from build123d import *

# Parameters (mm, degrees)
CYLINDER1016_R               = 1.5
CYLINDER1016_DEPTH           = 50
CYLINDER1016_PLACEMENT_ANGLE = 45
CYLINDER1012_R               = 1.5
CYLINDER1012_DEPTH           = 50
CYLINDER1012_PLACEMENT_ANGLE = 135
CYLINDER1014_R               = 1.5
CYLINDER1014_DEPTH           = 50
CYLINDER1017_R               = 1.5
CYLINDER1017_DEPTH           = 50
CYLINDER1017_PLACEMENT_ANGLE = 225
CYLINDER1018_R               = 1.5
CYLINDER1018_DEPTH           = 50
CYLINDER1013_R               = 1.5
CYLINDER1013_DEPTH           = 50
CYLINDER1013_PLACEMENT_ANGLE = 45
CYLINDER1015_R               = 1.5
CYLINDER1015_DEPTH           = 50
CYLINDER1011_R               = 52
CYLINDER1011_DEPTH           = 16
BOX416_W                     = 108
BOX416_H                     = 36
BOX416_DEPTH                 = 16


with BuildPart() as obj1:
    # Cylinder1016 → Cylinder1016 (new body)
    with BuildSketch(Plane.XY):
        Circle(CYLINDER1016_R)
    extrude(amount=CYLINDER1016_DEPTH)


with BuildPart() as obj1_1:
    # Cylinder1016 placement: moved
    add(obj1.part.moved(Location((39.59798, -39.59798, 2))).rotate(Axis((39.59798, -39.59798, 2), (0, 0, 1)), CYLINDER1016_PLACEMENT_ANGLE))


with BuildPart() as obj2:
    # Cylinder1012 → Cylinder1012 (new body)
    with BuildSketch(Plane.XY):
        Circle(CYLINDER1012_R)
    extrude(amount=CYLINDER1012_DEPTH)


with BuildPart() as obj2_1:
    # Cylinder1012 placement: moved
    add(obj2.part.moved(Location((39.59798, 39.59798, 2))).rotate(Axis((39.59798, 39.59798, 2), (0, 0, 1)), CYLINDER1012_PLACEMENT_ANGLE))


with BuildPart() as obj3:
    # Cylinder1014 → Cylinder1014 (new body)
    with BuildSketch(Plane(origin=(0, 56, 2), x_dir=(-1, 0, 0), z_dir=(0, 0, 1))):
        Circle(CYLINDER1014_R)
    extrude(amount=CYLINDER1014_DEPTH)


with BuildPart() as obj4:
    # Cylinder1017 → Cylinder1017 (new body)
    with BuildSketch(Plane.XY):
        Circle(CYLINDER1017_R)
    extrude(amount=CYLINDER1017_DEPTH)


with BuildPart() as obj4_1:
    # Cylinder1017 placement: moved
    add(obj4.part.moved(Location((-39.59798, 39.59798, 2))).rotate(Axis((-39.59798, 39.59798, 2), (0, 0, 1)), CYLINDER1017_PLACEMENT_ANGLE))


with BuildPart() as obj5:
    # Cylinder1018 → Cylinder1018 (new body)
    with BuildSketch(Plane(origin=(-56, 0, 2), x_dir=(0, -1, 0), z_dir=(0, 0, 1))):
        Circle(CYLINDER1018_R)
    extrude(amount=CYLINDER1018_DEPTH)


with BuildPart() as obj6:
    # Cylinder1013 → Cylinder1013 (new body)
    with BuildSketch(Plane.XY):
        Circle(CYLINDER1013_R)
    extrude(amount=CYLINDER1013_DEPTH)


with BuildPart() as obj6_1:
    # Cylinder1013 placement: moved
    add(obj6.part.moved(Location((-39.59798, -39.59798, 2))).rotate(Axis((-39.59798, -39.59798, 2), (0, 0, -1)), CYLINDER1013_PLACEMENT_ANGLE))


with BuildPart() as compound817:
    # Cylinder1015 → Cylinder1015 (new body)
    with BuildSketch(Plane(origin=(0, -56, 2), x_dir=(1, 0, 0), z_dir=(0, 0, 1))):
        Circle(CYLINDER1015_R)
    extrude(amount=CYLINDER1015_DEPTH)

    # Compound817: union obj1, obj2, obj3, obj4, obj5, obj6
    add(obj1_1.part)
    add(obj2_1.part)
    add(obj3.part)
    add(obj4_1.part)
    add(obj5.part)
    add(obj6_1.part)


with BuildPart() as obj7:
    # Cylinder1011 → Cylinder1011 (new body)
    with BuildSketch(Plane.XY.offset(20)):
        Circle(CYLINDER1011_R)
    extrude(amount=CYLINDER1011_DEPTH)


with BuildPart() as cut423:
    # Box416 → Box416 (new body)
    with BuildSketch(Plane(origin=(-54, -53, 20), x_dir=(1, 0, 0), z_dir=(0, 0, 1))):
        with Locations((54, 18)):
            Rectangle(BOX416_W, BOX416_H)
    extrude(amount=BOX416_DEPTH)

    # Cut424: cut obj7
    add(obj7.part, mode=Mode.SUBTRACT)


with BuildPart() as cut423_1:
    # Cut424 placement: moved
    add(cut423.part.moved(Location((0, 0, -10))))

    # Cut423: cut Compound817
    add(compound817.part, mode=Mode.SUBTRACT)


with BuildPart() as cut423_2:
    # Cut423 placement: moved
    add(cut423_1.part.moved(Location((0, 0, 6))))


solid = cut423_2.part
The model under review builds one solid part; all positions refer to its coordinate system, in mm. Coordinates: 2 decimals unless noted, no trailing zeros. Loops run counter-clockwise (first coordinate to the right, second up) from the corner with the lowest first, then second, coordinate; pieces in that order, holes last.
(1) Wall thickness on L1, parallel to X at y = -39.5, z = 23.5; L2, parallel to X at y = -19, z = 18; L3, parallel to X at y = -33.5, z = 18.25: over which ranges is each line inside the solid? List them lowest first.
Determined:
L1: x = -54 to -41.09, -38.1 to -33.82, 33.82 to 38.1, 41.09 to 54
L2: x = -54 to -48.4, 48.4 to 54
L3: x = -54 to -39.77, 39.77 to 54
(2) Consider section A-A, the plane y = -24. Give the boundary of the cut face in (x, z), plus the area to 3 significant figures.
Determined:
outline: (-54, 16) - (-46.13, 16) - (-46.13, 32) - (-54, 32) - close; (46.13, 16) - (54, 16) - (54, 32) - (46.13, 32) - close
area: 252 mm2
(3) Insertion check: P1, Ø2.5, axis at x = 39.6, y = -39.6, coming from the +Z side; P2, Ø1.5, axis at x = -8.5, z = 21.5, coming from the +Y side. Each pin has a flat end and moves straight along its axis. Give the tip position at first contact, or say it passes through.
Determined:
P1: passes through
P2: stops at y = -51.17
(4) Draft analysis for pull direction X (two halves, no side actions). For faces 1 (the flat face through (-13, -51, 32)), 2 (the cylindrical face through (-40.61, -38.49, 23.89)), 3 (the cylindrical face through (38.49, -40.61, 23.89)), 4 (the flat face through (54, -35, 24)), state which applies: +X half, -X half, draft (parallel to the pull), parting line (faces both ways), or undercut.
Determined:
face 1: draft
face 2: undercut
face 3: undercut
face 4: +X half
(5) Consider section B-B, the plane z = 27.25. Give the boundary of the cut face in (x, y), plus the area to 3 significant figures.
Determined:
outline: (-54, -53) - (54, -53) - (54, -17) - (49.14, -17) arc R52 cw to (-49.14, -17) - (-54, -17) - close; hole circle Ø3 at (-39.6, -39.6); hole circle Ø3 at (39.6, -39.6)
area: 1,360 mm2
(6) Consider section C-C, the plane y = -50.5. Give the boundary of the cut face in (x, z), plus the area to 3 significant figures.
Determined:
outline: (-54, 16) - (-12.4, 16) - (-12.4, 32) - (-54, 32) - close; (12.4, 16) - (54, 16) - (54, 32) - (12.4, 32) - close
area: 1,330 mm2
(7) Consider section D-D, the plane x = 5. Give the boundary of the cut face in (y, z), plus the area to 3 significant figures.
Determined:
outline: (-53, 16) - (-51.76, 16) - (-51.76, 32) - (-53, 32) - close
area: 19.9 mm2
